Autodesk Inventor part; units mm, degrees
ref_plane "YZ Plane" through (0, 0, 0) normal (1, 0, 0) x (0, 1, 0)
ref_plane "XZ Plane" through (0, 0, 0) normal (0, 1, 0) x (-1, 0, 0)
ref_plane "XY Plane" through (0, 0, 0) normal (0, 0, 1) x (1, 0, 0)
sketch "Sketch1" plane through (0, 0, 0) normal (0, 1, 0) x (-1, 0, 0)
  line L0 (31.575, 38.95) -> (-5.625, 38.95)
  line L1 (-5.625, 38.95) -> (-33.925, -36.6)
  line L2 (-33.925, -36.6) -> (-28.075, -42.45)
  line L3 (-28.075, -42.45) -> (28.075, -42.45)
  line L4 (28.075, -42.45) -> (31.575, -38.95)
  line L5 (31.575, -38.95) -> (31.575, 38.95)
  point P0 (0, 0)
  point P1 (0, -42.45)
  point P2 (31.575, 0)
  dimension "d0" = 3.5
  dimension "d1" = 3.5
  dimension "d2" = 81.4
  dimension "d3" = 37.2
  dimension "d4" = 65.5
  dimension "d5" = 59.65
extrude "Extrusion1" add sketch "Sketch1" along normal mid plane 1.7
equation "\"d1\" = d0"
properties part number "StrategyCard_Single" material "Paper"
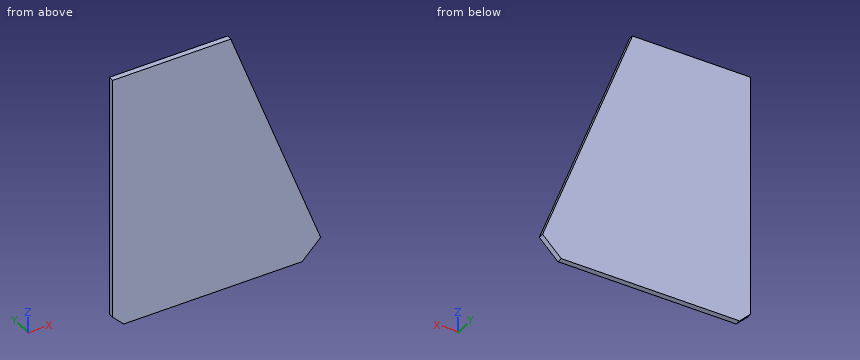
The listing builds one solid part. Answer for the finished solid, in the listing's coordinates (mm). Give positions to 0.01 mm unless a question says otherwise; leave off trailing zeros. Loops run counter-clockwise (first coordinate to the right, second up) from the corner with the lowest first, then second, coordinate; pieces in that order, holes last. Notation, with made-up numbers: (56.5, 29) - (68.5, 29) arc R20 cw to (68.5, 50) - close; hole circle Ø4 at (10, 8.25). An arc over 180 degrees is marked (long way). Return JSON: item names as keys, results as strings. Group by question number.
1. Straight lines are drawn through the part: line 1 (X direction, y = -0.6, z = 7.5) (3 decimals); line 2 (X direction, y = -0.45, z = 30) (3 decimals); line 3 (Z direction, x = -29, y = 0.25) (3 decimals). For each, find the intervals that lie inside material, in ascending order. Write a range as [from, to].
2. Find section C-C (z = -31). Write down the section's boundary in (x, y) (3 decimals).
3. Find section A-A (y = 0.15). Write down the section's boundary in (x, z) (3 decimals).
4. Given pin 1 Ø1 at (y, z) = (0, 16.5) entering from +X, flat-ended and moving along its own axis, determine where the tip first touches the part or whether it passes through.
5. Find section B-B (x = 27). Write down the section's boundary in (y, z), then the cut area to 3 significant figures.
Verdict:
{
 "1": {"line 1": "x = [-31.575, 17.406]", "line 2": "x = [-31.575, 8.978]", "line 3": "z = [-41.525, 38.95]"},
 "2": {"outline": "(-31.575, -0.85) - (31.827, -0.85) - (31.827, 0.85) - (-31.575, 0.85) - close"},
 "3": {"outline": "(-31.575, -38.95) - (-28.075, -42.45) - (28.075, -42.45) - (33.925, -36.6) - (5.625, 38.95) - (-31.575, 38.95) - close"},
 "4": {"pin 1": "stops at x = 14.22"},
 "5": {"outline": "(-0.85, -42.45) - (0.85, -42.45) - (0.85, -18.11) - (-0.85, -18.11) - close", "area": "41.4 mm^2"}
}
